Autodesk Fusion 360 part; units mm, degrees
sketch "Sketch1" plane through (0, 0, 0) normal (1, 0, 0) x (0, 0, -1)
  line L0 (-50, 20) -> (-4, 20)
  line L1 (-4, 20) -> (-4, -11.5)
  line L2 (-4, -11.5) -> (-50, -11.5)
  line L3 (-50, -11.5) -> (-50, 20)
  line L4 (-65.5096, 6.4803) -> (-1.0096, 6.4803)
  line L5 (-1.0096, 6.4803) -> (-1.0096, -9.308)
  line L6 (-1.0096, -9.308) -> (-65.5096, -9.308)
  line L7 (-65.5096, -9.308) -> (-65.5096, 6.4803)
  line L8 (52, 50) -> (64.5, 50)
  line L9 (65.5, 49) -> (65.5, 45.5)
  line L10 (65.5, 45.5) -> (51, 45.5)
  line L11 (51, 45.5) -> (51, 49)
  line L12 (51, 45.5) -> (55.5, 45.5)
  line L13 (55.5, 45.5) -> (55.5, 39)
  line L14 (54.5, 38) -> (52, 38)
  line L15 (51, 39) -> (51, 45.5)
  line L16 (65.5, 45.5) -> (61, 45.5)
  line L17 (61, 45.5) -> (61, 19.5)
  line L18 (61, 19.5) -> (65.5, 19.5)
  line L19 (65.5, 19.5) -> (65.5, 45.5)
  line L20 (65.5, 19.5) -> (54.5, 19.5)
  line L21 (53.5, 18.5) -> (53.5, 16)
  line L22 (54.5, 15) -> (65.5, 15)
  line L23 (65.5, 15) -> (65.5, 19.5)
  line L24 (65.5, 15) -> (75.5, 15)
  line L25 (75.5, 15) -> (75.5, 25.5)
  line L26 (74.5, 26.5) -> (65.5, 26.5)
  line L27 (65.5, 26.5) -> (65.5, 15)
  line L28 (75.5, 15) -> (85, 15)
  line L29 (86, 16) -> (86, 19.5)
  line L30 (86, 19.5) -> (75.5, 19.5)
  line L31 (75.5, 19.5) -> (75.5, 15)
  line L32 (86, 19.5) -> (81.5, 19.5)
  line L33 (81.5, 19.5) -> (81.5, 25.5)
  line L34 (82.5, 26.5) -> (85, 26.5)
  line L35 (86, 25.5) -> (86, 19.5)
  arc A0 (52, 50) -> (51, 49) centre (52, 49) ccw
  arc A1 (65.5, 49) -> (64.5, 50) centre (64.5, 49) ccw
  arc A2 (51, 39) -> (52, 38) centre (52, 39) ccw
  arc A3 (54.5, 38) -> (55.5, 39) centre (54.5, 39) ccw
  arc A4 (54.5, 19.5) -> (53.5, 18.5) centre (54.5, 18.5) ccw
  arc A5 (53.5, 16) -> (54.5, 15) centre (54.5, 16) ccw
  arc A6 (75.5, 25.5) -> (74.5, 26.5) centre (74.5, 25.5) ccw
  arc A7 (82.5, 26.5) -> (81.5, 25.5) centre (82.5, 25.5) ccw
  arc A8 (86, 25.5) -> (85, 26.5) centre (85, 25.5) ccw
  arc A9 (85, 15) -> (86, 16) centre (85, 16) ccw
  point P0 (51, 50)
  point P1 (65.5, 50)
  point P2 (51, 38)
  point P3 (53.5, 19.5)
  point P4 (86, 15)
  point P5 (86, 26.5)
  dimension "d1" = 46
  dimension "d2" = 31.5
  dimension "d3" = 64.5
  dimension "d4" = 14.5
  dimension "d5" = 4.5
  dimension "d6" = 4.5
  dimension "d7" = 7.5
  dimension "d8" = 4.5
  dimension "d9" = 26
  dimension "d10" = 12
  dimension "d11" = 4.5
  dimension "d12" = 10
  dimension "d13" = 11.5
  dimension "d14" = 10.5
  dimension "d15" = 4.5
  dimension "d16" = 4.5
  dimension "d17" = 7
  dimension "d18" = 1
extrude "Extrude1" add sketch "Sketch1" along normal blind 4.5 contours L8 L9 L10 L11 L12 L16 A0 A1 | L10 L12 L13 L14 L15 A2 A3 | L10 L16 L17 L18 L19 L20 L27 | L19 L23 L24 L25 L26 L27 L31 A6 | L18 L20 L21 L22 L23 L27 A4 A5 | L25 L28 L29 L30 L31 L32 A9 | L30 L32 L33 L34 L35 A7 A8
fillet "Fillet1" radius 1 26 edges at (4.5, 37.75, -65.5) (4.5, 49.7071, -65.2071) (4.5, 50, -58.25) (4.5, 49.7071, -51.2929) (4.5, 44, -51) (4.5, 38.2929, -51.2929) (4.5, 38, -53.25) (4.5, 38.2929, -55.2071) (4.5, 42.25, -55.5) (4.5, 22.5, -75.5) (4.5, 26.2071, -75.2071) (4.5, 26.5, -70) (4.5, 19.5, -78.5) (4.5, 19.5, -57.75) (4.5, 19.2071, -53.7929) (4.5, 17.25, -53.5) (4.5, 15.2929, -53.7929) (4.5, 15, -69.75) (4.5, 15.2929, -85.7071) (4.5, 20.75, -86) (4.5, 26.2071, -85.7071) (4.5, 26.5, -83.75) (4.5, 26.2071, -81.7929) (4.5, 22.5, -81.5) (4.5, 32.5, -61) (4.5, 45.5, -58.25)
fillet "Fillet2" radius 1 26 edges at (0, 22.5, -75.5) (0, 26.2071, -75.2071) (0, 26.5, -70) (0, 37.75, -65.5) (0, 49.7071, -65.2071) (0, 50, -58.25) (0, 49.7071, -51.2929) (0, 44, -51) (0, 38.2929, -51.2929) (0, 38, -53.25) (0, 38.2929, -55.2071) (0, 42.25, -55.5) (0, 45.5, -58.25) (0, 32.5, -61) (0, 19.5, -57.75) (0, 19.2071, -53.7929) (0, 17.25, -53.5) (0, 15.2929, -53.7929) (0, 15, -69.75) (0, 15.2929, -85.7071) (0, 20.75, -86) (0, 26.2071, -85.7071) (0, 26.5, -83.75) (0, 26.2071, -81.7929) (0, 22.5, -81.5) (0, 19.5, -78.5)
equation "d4 = 4.5 mm + 5.5 mm + 4.5 mm"
equation "d7 = 12 mm - d5"
equation "d10 = 4.5 mm + 7.5 mm"
equation "d12 = 5.5 mm + 4.5 mm"
equation "d13 = 4.5 mm + 7 mm"
equation "d14 = 6 mm + 4.5 mm"
The listing builds one solid part. Answer for the finished solid, in the listing's coordinates (mm). A direction names the side the tool comes from. Round coordinates to 2 decimals unless told otherwise and drop trailing zeros. Loops run counter-clockwise (first coordinate to the right, second up) from the corner with the lowest first, then second, coordinate; pieces in that order, holes last.
Q1. Section A-A, the plane z = -60 is taken. Determine the outline of the cut face in (x, y), then the cut area to 3 significant figures.
Q2. For a pull along Y with two mould halves and no side action, classify faces 1 (the face through (4.215, 19.199, -78.444)), 2 (the face through (0.285, 37.085, -65.199)), 3 (the face through (0.285, 45.801, -58.198)) as released by +Y, released by -Y, zero draft, split by the parting line, or undercut.
Q3. Section D-D, the plane y = 47.5 is taken. Determine the outline of the cut face in (x, z), then the cut area to 3 significant figures.
Q4. Section B-B, the plane y = 21 is taken. Determine the outline of the cut face in (x, z), then the cut area to 3 significant figures.
Q5. Which of the six approach directions +Z, -Z, +X, -X, +Y, -Y give full straight-line access (tool end or side, diameter ignored) to faces 4 (the face through (0.301, 26.215, -83.732)), 5 (the face through (4.215, 26.199, -83.732)), 6 (the face through (4.215, 19.199, -58.198))?
Q6. Section C-C, the plane x = 2.2 is taken. Determine the outline of the cut face in (y, z).
Q7. Given pin 1 Ø2 at (x, z) = (2.5, -71.5) entering from +Y; pin 2 Ø1.2 at (x, y) = (2, 42.5) entering from -Z; pin 3 Ø1.2 at (x, y) = (2.5, 17.5) entering from +Z, each flat-ended and moving along its own axis, determine where each tip first touches the part or whether it passes through.
Q8. Find the intervals of material crossed by line 1 (Z direction, x = 3.05, y = 43); line 2 (Z direction, x = 3.05, y = 36.5); line 3 (Y direction, x = 1.55, z = -56), in increasing order.
Completed:
1. outline: (0, 16) arc R1 ccw to (1, 15) - (3.5, 15) arc R1 ccw to (4.5, 16) - (4.5, 18.5) arc R1 ccw to (3.5, 19.5) - (1, 19.5) arc R1 ccw to (0, 18.5) - close; (0, 46.5) arc R1 ccw to (1, 45.5) - (3.5, 45.5) arc R1 ccw to (4.5, 46.5) - (4.5, 49) arc R1 ccw to (3.5, 50) - (1, 50) arc R1 ccw to (0, 49) - close
1. area: 38.8 mm2
2. face 1: released by +Y
2. face 2: zero draft
2. face 3: undercut
3. outline: (0, -64.5) arc R1 ccw to (1, -65.5) - (3.5, -65.5) arc R1 ccw to (4.5, -64.5) - (4.5, -52) arc R1 ccw to (3.5, -51) - (1, -51) arc R1 ccw to (0, -52) - close
3. area: 64.4 mm2
4. outline: (0, -85) arc R1 ccw to (1, -86) - (3.5, -86) arc R1 ccw to (4.5, -85) - (4.5, -82.5) arc R1 ccw to (3.5, -81.5) - (1, -81.5) arc R1 ccw to (0, -82.5) - close; (0, -74.5) arc R1 ccw to (1, -75.5) - (3.5, -75.5) arc R1 ccw to (4.5, -74.5) - (4.5, -62) arc R1 ccw to (3.5, -61) - (1, -61) arc R1 ccw to (0, -62) - close
4. area: 83.8 mm2
5. face 4: -Z, -X, +Y
5. face 5: -Z, +X, +Y
5. face 6: +Z, +X
6. outline: (15, -85) arc R1 ccw to (16, -86) - (25.5, -86) arc R1 ccw to (26.5, -85) - (26.5, -82.5) arc R1 ccw to (25.5, -81.5) - (19.5, -81.5) - (19.5, -75.5) - (25.5, -75.5) arc R1 ccw to (26.5, -74.5) - (26.5, -65.5) - (49, -65.5) arc R1 ccw to (50, -64.5) - (50, -52) arc R1 ccw to (49, -51) - (39, -51) arc R1 ccw to (38, -52) - (38, -54.5) arc R1 ccw to (39, -55.5) - (45.5, -55.5) - (45.5, -61) - (19.5, -61) - (19.5, -54.5) arc R1 ccw to (18.5, -53.5) - (16, -53.5) arc R1 ccw to (15, -54.5) - close
7. pin 1: stops at y = 26.5
7. pin 2: stops at z = -65.5
7. pin 3: stops at z = -53.5
8. line 1: z = -65.5 to -61, -55.5 to -51
8. line 2: z = -65.5 to -61
8. line 3: y = 15 to 19.5, 45.5 to 50
